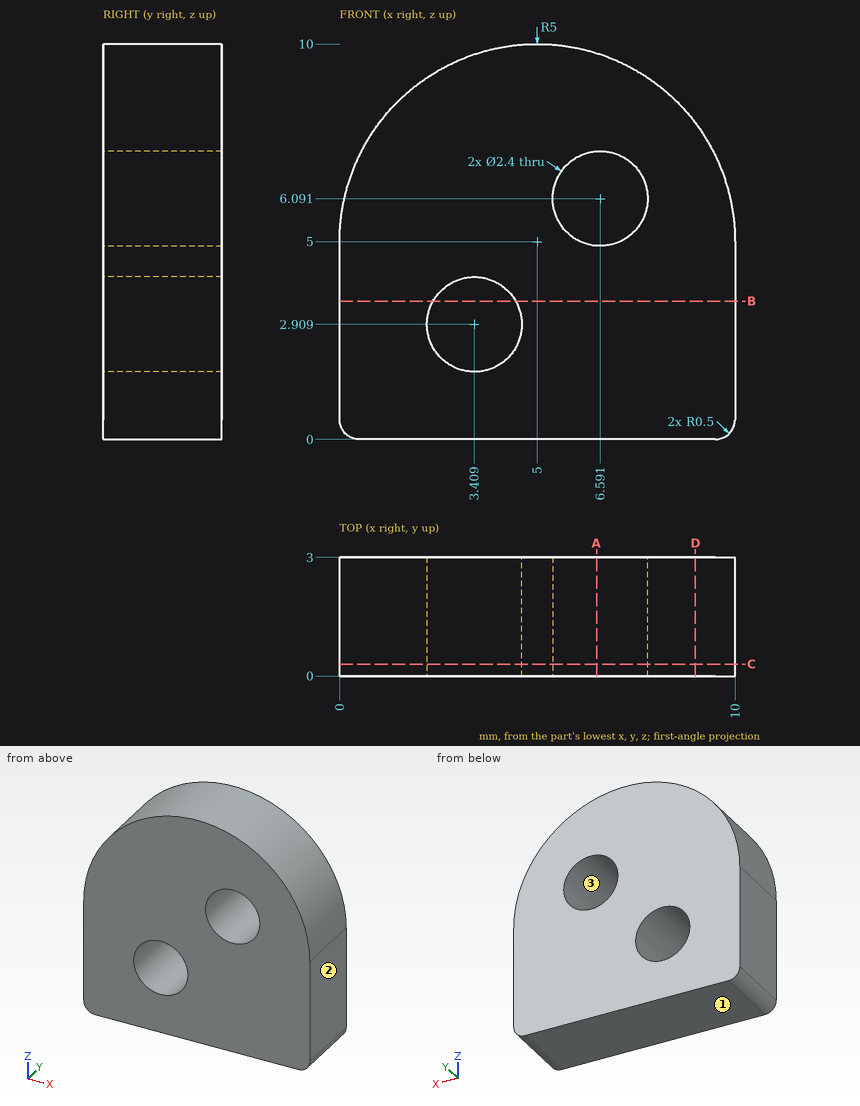
Check sheet for the drawn part. Datum: minimum x, y, z corner. Units: mm. Round coordinates to 2 decimals unless told otherwise and drop trailing zeros. Write each loop counter-clockwise with the first axis right and the second up, starting at its lowest first coordinate (ties: lowest second). Pieces come first, ordered by that corner, then holes. Notation, with made-up numbers: (85, 64.25) -> (138, 64.25) arc R28 ccw to (138, 90.25) -> close; hole circle Ø8 at (8.5, 50). An arc over 180 degrees is marked (long way). Write each question's results on one line, items separated by ' | '. Start each with the question number.
1. Cross-section at A-A (x = 6.5). Enter the section's corners in (y, z).
2. Cross-section at B-B (z = 3.5). Enter the section's corners in (x, y), then the cut area to 3 significant figures.
3. Draft check along X on the marked faces 1, 2 and 3. Enter one of: +X half, -X half, draft (parallel to the pull), parting line (faces both ways), or undercut.
4. Depth check by flat-ended pin: P1, Ø1.5, axis at x = 6.5, y = 2, coming from the +Z side. Enter the tip coordinate at first touch or a pass-through.
5. Cross-section at D-D (x = 9). Enter the section's corners in (y, z), then the cut area to 3 significant figures.
6. Material ranges on probe 1 along X at (y, z) = (2.25, 6.5); probe 2 along Z at (x, y) = (6.25, 2.15); probe 3 along Z at (x, y) = (3.75, 2), recorded low to high. Write a range as from..to.
7. Cross-section at C-C (y = 0.3). Enter the section's corners in (x, z).
Solutions:
1) outline: (0, 0) -> (3, 0) -> (3, 4.89) -> (0, 4.89) -> close; (0, 7.29) -> (3, 7.29) -> (3, 9.77) -> (0, 9.77) -> close
2) outline: (0, 0) -> (2.36, 0) -> (2.36, 3) -> (0, 3) -> close; (4.45, 0) -> (10, 0) -> (10, 3) -> (4.45, 3) -> close | area: 23.7 mm2
3) face 1: draft | face 2: +X half | face 3: undercut
4) P1: stops at z = 9.94
5) outline: (0, 0) -> (3, 0) -> (3, 8) -> (0, 8) -> close | area: 24.0 mm2
6) probe 1: x = 0.23..5.46, 7.72..9.77 | probe 2: z = 0..4.94, 7.24..9.84 | probe 3: z = 0..1.76, 4.06..9.84
7) outline: (0, 0.5) arc R0.5 ccw to (0.5, 0) -> (9.5, 0) arc R0.5 ccw to (10, 0.5) -> (10, 5) arc R5 ccw to (0, 5) -> close; hole circle Ø2.4 at (3.41, 2.91); hole circle Ø2.4 at (6.59, 6.09)
